Here's how the part is built. I have some questions about the finished solid (model axes, mm). A direction names the side the tool comes from. Coordinates: 2 decimals unless noted, no trailing zeros. Loops run counter-clockwise (first coordinate to the right, second up) from the corner with the lowest first, then second, coordinate; pieces in that order, holes last. Notation, with made-up numbers: M 63,-16.5 L 91,-16.5 A18 cw 91,14.5 Z; hole C 48,56 d7. An arc over 180 degrees is marked long. Use CSV: the item, a comma, the result in double quotes. Start each with the question number.
Q1. If we section it at C-C (y = -79): Please give me the cut outline in (x, z), and give its area (3 significant figures).
Q2. Which directions (+Z, -Z, +X, -X, +Y, -Y) give clear straight access to the entire face, cutting with the end or side of a thin tool? Please do faces 1 (the flat face through (-52, -136.802, 19)), 2 (the cylindrical face through (-99.73, -2.85, 4.93)), 3 (the flat face through (-51, -135.877, 1)), 4 (the cylindrical face through (-49.34, -137.3, 12.79)), 5 (the flat face through (-15, -46, 3)).
Q3. Please list where these lines run through material, in increasing order: probe 1 along Y at (x, z) = (-20, 5.5); probe 2 along Y at (x, z) = (-49, 15.5); probe 3 along Z at (x, y) = (-33, -122.5). Write a range as [from, to].
Q4. If we section it at D-D (y = -46.5): Please give me the cut outline in (x, z), and give its area (3 significant figures).
Q5. For pin 1 Ø3 at (x, y) = (-21.5, -126) entering from +Z; pin 2 Ø11 at (x, y) = (-24, -42) entering from +Z; pin 3 Ø7 at (x, z) = (-10, 20) entering from +Y, each with a flat end and sliding along its axis, tell me the tip position at first contact or that it passes through.
Q6. If we section it at A-A (z = 20): Please give me the cut outline in (x, y) (3 decimals), and give its area (3 significant figures).
Q7. If we mould it in two halves opening along Z, with no side actions, what happens to faces 6 (the cylindrical face through (-93.778, -19.514, 6.451)), 7 (the flat face through (-80, -25, 3)), 8 (the flat face through (-52, -54, 0)), 9 (the cylindrical face through (-10, -137, 17))? For each: +Z half, -Z half, draft (parallel to the pull), parting line (faces both ways), or undercut.
Q8. If we section it at B-B (y = -20): Please give me the cut outline in (x, z), and give its area (3 significant figures).
from build123d import *

# Parameters (mm, degrees)
SKETCH2_R           = 11.05
BOSS_EXTRUDE2_DEPTH = 10
SKETCH2_4_R         = 11.05
SKETCH2_4_R_2       = 5
BOSS_EXTRUDE3_DEPTH = 3
SKETCH4_R           = 1.6
CUT_EXTRUDE3_DEPTH  = 10
SKETCH4_5_R         = 3
SKETCH4_5_R_2       = 1.6
CUT_EXTRUDE4_DEPTH  = 3
SKETCH5_W           = 92.15
SKETCH5_H           = 21.15
SKETCH5_W_2         = 87.95
SKETCH5_H_2         = 16.95
CUT_EXTRUDE5_DEPTH  = 3
SKETCH6_W           = 102.73844499
SKETCH6_H           = 25
BOSS_EXTRUDE4_DEPTH = 5
SKETCH7_R           = 1.575
CUT_EXTRUDE6_DEPTH  = 5
SKETCH7_3_R         = 3
SKETCH7_3_R_2       = 1.575
CUT_EXTRUDE7_DEPTH  = 1


with BuildPart() as part:
    # Sketch2 → Boss-Extrude2 (new body)
    with BuildSketch(Plane.XY):
        with BuildLine():
            Line((-10, 0), (-92.73844499, 0))
            ThreePointArc((-92.73844499, 0), (-99.809512802, -2.928932188), (-102.73844499, -10))
            Line((-102.73844499, -10), (-102.73844499, -141.80223365))
            Line((-102.73844499, -141.80223365), (0, -141.80223365))
            Line((0, -141.80223365), (0, -10))
            ThreePointArc((0, -10), (-2.928932188, -2.928932188), (-10, 0))
        make_face()
        with Locations((-82.73844499, -20)):
            Circle(SKETCH2_R, mode=Mode.SUBTRACT)
        with Locations((-20, -43.89848365)):
            Circle(SKETCH2_R, mode=Mode.SUBTRACT)
    extrude(amount=BOSS_EXTRUDE2_DEPTH)

    # Sketch2_4 → Boss-Extrude3 (add)
    # profile 1 of 2: a face of its own
    with BuildSketch(Plane.XY):
        with Locations((-82.73844499, -20)):
            Circle(SKETCH2_4_R)
        with Locations((-82.73844499, -20)):
            Circle(SKETCH2_4_R_2, mode=Mode.SUBTRACT)
    # profile 2 of 2: a face of its own
    with BuildSketch(Plane.XY):
        with Locations((-20, -43.89848365)):
            Circle(SKETCH2_4_R)
        with Locations((-20, -43.89848365)):
            Circle(SKETCH2_4_R_2, mode=Mode.SUBTRACT)
    extrude(amount=BOSS_EXTRUDE3_DEPTH)

    # Sketch4 → Cut-Extrude3 (cut)
    with BuildSketch(Plane.XY.offset(10)):
        with Locations((-82.19075699, -127.45223365)):
            Circle(SKETCH4_R)
        with Locations((-61.64306899, -127.45223365)):
            Circle(SKETCH4_R)
        with Locations((-41.09538099, -127.45223365)):
            Circle(SKETCH4_R)
        with Locations((-20.54769299, -127.45223365)):
            Circle(SKETCH4_R)
    extrude(amount=-CUT_EXTRUDE3_DEPTH, mode=Mode.SUBTRACT)

    # Sketch4_5 → Cut-Extrude4 (cut)
    # profile 1 of 4: a face of its own
    with BuildSketch(Plane.XY.offset(10)):
        with Locations((-82.19075699, -127.45223365)):
            Circle(SKETCH4_5_R)
        with Locations((-82.19075699, -127.45223365)):
            Circle(SKETCH4_5_R_2, mode=Mode.SUBTRACT)
    # profile 2 of 4: a face of its own
    with BuildSketch(Plane.XY.offset(10)):
        with Locations((-61.64306899, -127.45223365)):
            Circle(SKETCH4_5_R)
        with Locations((-61.64306899, -127.45223365)):
            Circle(SKETCH4_5_R_2, mode=Mode.SUBTRACT)
    # profile 3 of 4: a face of its own
    with BuildSketch(Plane.XY.offset(10)):
        with Locations((-41.09538099, -127.45223365)):
            Circle(SKETCH4_5_R)
        with Locations((-41.09538099, -127.45223365)):
            Circle(SKETCH4_5_R_2, mode=Mode.SUBTRACT)
    # profile 4 of 4: a face of its own
    with BuildSketch(Plane.XY.offset(10)):
        with Locations((-20.54769299, -127.45223365)):
            Circle(SKETCH4_5_R)
        with Locations((-20.54769299, -127.45223365)):
            Circle(SKETCH4_5_R_2, mode=Mode.SUBTRACT)
    extrude(amount=-CUT_EXTRUDE4_DEPTH, mode=Mode.SUBTRACT)

    # Sketch5 → Cut-Extrude5 (cut)
    with BuildSketch(Plane(origin=(0, 0, 0), x_dir=(-1, 0, 0), z_dir=(0, 0, -1))):
        with Locations((51.369222495, -127.40223365)):
            Rectangle(SKETCH5_W, SKETCH5_H)
        with Locations((51.369222495, -127.40223365)):
            Rectangle(SKETCH5_W_2, SKETCH5_H_2, mode=Mode.SUBTRACT)
    extrude(amount=-CUT_EXTRUDE5_DEPTH, mode=Mode.SUBTRACT)

    # Sketch6 → Boss-Extrude4 (add)
    with BuildSketch(Plane.XZ.offset(141.80223365)):
        with Locations((-51.369222495, 12.5)):
            Rectangle(SKETCH6_W, SKETCH6_H)
    extrude(amount=-BOSS_EXTRUDE4_DEPTH)

    # Sketch7 → Cut-Extrude6 (cut)
    with BuildSketch(Plane(origin=(0, -136.80223365, 0), x_dir=(1, 0, 0), z_dir=(0, 1, 0))):
        with Locations(Location((-92.73844499, -20, 0), (0, 0, 270))):
            Circle(SKETCH7_R)
        with Locations(Location((-51.369222495, -15, 0), (0, 0, 270))):
            Circle(SKETCH7_R)
        with Locations(Location((-10, -20, 0), (0, 0, 270))):
            Circle(SKETCH7_R)
    extrude(amount=-CUT_EXTRUDE6_DEPTH, mode=Mode.SUBTRACT)

    # Sketch7_3 → Cut-Extrude7 (cut)
    # profile 1 of 3: a face of its own
    with BuildSketch(Plane(origin=(0, -136.80223365, 0), x_dir=(1, 0, 0), z_dir=(0, 1, 0))):
        with Locations(Location((-92.73844499, -20, 0), (0, 0, 270))):
            Circle(SKETCH7_3_R)
        with Locations(Location((-92.73844499, -20, 0), (0, 0, 270))):
            Circle(SKETCH7_3_R_2, mode=Mode.SUBTRACT)
    # profile 2 of 3: a face of its own
    with BuildSketch(Plane(origin=(0, -136.80223365, 0), x_dir=(1, 0, 0), z_dir=(0, 1, 0))):
        with Locations(Location((-51.369222495, -15, 0), (0, 0, 270))):
            Circle(SKETCH7_3_R)
        with Locations(Location((-51.369222495, -15, 0), (0, 0, 270))):
            Circle(SKETCH7_3_R_2, mode=Mode.SUBTRACT)
    # profile 3 of 3: a face of its own
    with BuildSketch(Plane(origin=(0, -136.80223365, 0), x_dir=(1, 0, 0), z_dir=(0, 1, 0))):
        with Locations(Location((-10, -20, 0), (0, 0, 270))):
            Circle(SKETCH7_3_R)
        with Locations(Location((-10, -20, 0), (0, 0, 270))):
            Circle(SKETCH7_3_R_2, mode=Mode.SUBTRACT)
    extrude(amount=-CUT_EXTRUDE7_DEPTH, mode=Mode.SUBTRACT)


solid = part.part
Results below:
1,outline,"M -102.74,0 L 0,0 L 0,10 L -102.74,10 Z"
1,area,"1,030 mm^2"
2,face 1,"+Z, +X, -X, +Y"
2,face 2,"+Z, -Z, -X, +Y"
2,face 3,"-Z"
2,face 4,"+Y"
2,face 5,"+Z"
3,probe 1,"[-141.8, -128.96], [-125.95, -54.95], [-32.85, 0]"
3,probe 2,"[-141.8, -137.8]"
3,probe 3,"[0, 10]"
4,outline,"M -102.74,0 L -24.27,0 L -24.27,3 L -30.74,3 L -30.74,10 L -102.74,10 Z; M -15.73,0 L 0,0 L 0,10 L -9.26,10 L -9.26,3 L -15.73,3 Z"
4,area,"851 mm^2"
5,pin 1,"z = 10"
5,pin 2,"z = 3"
5,pin 3,"y = -136.8"
6,outline,"M -102.738,-141.802 L -94.313,-141.802 L -94.313,-137.802 L -95.738,-137.802 L -95.738,-136.802 L -102.738,-136.802 Z; M -91.163,-141.802 L -11.575,-141.802 L -11.575,-137.802 L -13,-137.802 L -13,-136.802 L -89.738,-136.802 L -89.738,-137.802 L -91.163,-137.802 Z; M -8.425,-141.802 L 0,-141.802 L 0,-136.802 L -7,-136.802 L -7,-137.802 L -8.425,-137.802 Z"
6,area,"476 mm^2"
7,face 6,"draft"
7,face 7,"+Z half"
7,face 8,"-Z half"
7,face 9,"undercut"
8,outline,"M -102.74,0 L -87.74,0 L -87.74,3 L -93.79,3 L -93.79,10 L -102.74,10 Z; M -77.74,0 L 0,0 L 0,10 L -71.69,10 L -71.69,3 L -77.74,3 Z"
8,area,"843 mm^2"
